from build123d import *


with BuildPart() as part:
    # Sketch1 → Revolve1 (revolve)
    with BuildSketch(Plane(origin=(0, 0, 0), x_dir=(0, 0, -1), z_dir=(1, 0, 0))):
        with BuildLine():
            Line((39.02588692, 15.407979857), (43.460514917, 27.592020143))
            ThreePointArc((43.460514917, 27.592020143), (43.826631102, 28.069152044), (44.400207538, 28.25))
            Line((44.400207538, 28.25), (53.3, 28.25))
            Line((53.3, 28.25), (53.3, 24.25))
            ThreePointArc((53.3, 24.25), (58.661988488, 12.648147098), (60.5, 0))
            Line((60.5, 0), (0, 0))
            Line((0, 0), (0, 11.2))
            Line((0, 11.2), (8.3, 11.2))
            Line((8.3, 11.2), (8.3, 14.75))
            Line((8.3, 14.75), (38.086194299, 14.75))
            ThreePointArc((38.086194299, 14.75), (38.659770736, 14.930847956), (39.02588692, 15.407979857))
        make_face()
    revolve(axis=Axis((0, 0, 0), (0, 0, -1)))


solid = part.part
Verification items for the finished model (mm, model axes). A direction names the side the tool comes from. Give positions to 0.01 mm unless a question says otherwise; leave off trailing zeros. Write each loop counter-clockwise with the first axis right and the second up, starting at its lowest first coordinate (ties: lowest second). Pieces come first, ordered by that corner, then holes.
(1) Cross-section at A-A (x = 0). Enter the section's corners in (y, z).
(2) Cross-section at C-C (z = -17). Enter the section's corners in (x, y), plus the area to 3 significant figures.
(3) Cross-section at D-D (z = -55). Enter the section's corners in (x, y).
(4) Access from +Z, -Z, +X, -X, +Y, -Y to the whole of each face (thin tool, end or side, straight path). Record for faces 1 (the face through (21.1, 12.4, -53.3)), 2 (the face through (4.43, 14.07, -23.4)), 3 (the face through (0, 0, 0)).
(5) Gauge pin test, flat ends, axial feed: pin 1 (17 mm diameter, centred on x = 3, y = 9.5, fed in from -Z); pin 2 (9 mm diameter, centred on x = 7, y = 2.5, fed in from +Z); pin 3 (12 mm diameter, centred on x = -22, y = -9.5, fed in from -Z); pin 4 (5 mm diameter, centred on y = -14.5, z = -7, fed in from +X). Record the tip position at first contact, or that the pin passes through.
(6) Material ranges on line 1 (Z direction, x = 24, y = 13.5); line 2 (Z direction, x = -16, y = 3); line 3 (X direction, y = 13, z = -15.5), recorded low to high.
Worked out:
1. outline: (-28.25, -53.3) - (-24.25, -53.3) arc R44.44 ccw to (24.25, -53.3) - (28.25, -53.3) - (28.25, -44.4) arc R1 ccw to (27.59, -43.46) - (15.41, -39.03) arc R1 cw to (14.75, -38.09) - (14.75, -8.3) - (11.2, -8.3) - (11.2, 0) - (-11.2, 0) - (-11.2, -8.3) - (-14.75, -8.3) - (-14.75, -38.09) arc R1 cw to (-15.41, -39.03) - (-27.59, -43.46) arc R1 ccw to (-28.25, -44.4) - close
2. outline: circle Ø29.5 at (0, 0)
2. area: 683 mm2
3. outline: circle Ø42.83 at (0, 0)
4. face 1: -Z
4. face 2: +Z
4. face 3: +Z, +X, -X, +Y, -Y
5. pin 1: stops at z = -60.48
5. pin 2: stops at z = 0
5. pin 3: stops at z = -56.71
5. pin 4: stops at x = 8.04
6. line 1: z = -53.3 to -43.44
6. line 2: z = -57.41 to -39.34
6. line 3: x = -6.97 to 6.97
